The model under review builds one solid part; all positions refer to its coordinate system, in mm. A direction names the side the tool comes from. Coordinates: 2 decimals unless noted, no trailing zeros. Order: outer loops, then holes, each group sorted by start corner. A loop starts at its lowest first (then second) coordinate and runs counter-clockwise, first axis right, second up. Notation, with made-up numbers: (6, -6) -> (64, -6) arc R32 ccw to (64, 20) -> close; hole circle Ø9 at (-16.75, -18.5). An arc over 180 degrees is marked (long way). Use one line per item in the form item = value.
from build123d import *

# Parameters (mm, degrees)
HUB_DEPTH                         = 14
SKETCH4_R                         = 6
ARM_INSERT_1_DEPTH                = 30
SKETCH5_R                         = 6
ARM_INSERT_2_DEPTH                = 30
ARM_START                         = 30
SKETCH6_R                         = 6
ARM_INSERT_3_DEPTH                = 30
SKETCH7_R                         = 6
ARM_INSERT_4_DEPTH                = 30
SKETCH8_R                         = 8
HUB_LIGHTENING_HOLE_DEPTH         = 64.878932647
SKETCH9_R                         = 2.5
ARM_1_AND_3_LIGHTENING_HOLE_DEPTH = 100.535396168
SKETCH10_R                        = 2.5
ARM_2_AND_4_LIGHTENING_HOLE_DEPTH = 100.535396227


with BuildPart() as part:
    # Sketch1 → Hub (new body)
    with BuildSketch(Plane(origin=(0, 0, 0), x_dir=(1, 0, 0), z_dir=(0, 1, 0))):
        Polygon((14.071067812, 7), (14.071067812, -7), (7, -14.071067812), (-7, -14.071067812), (-14.071067812, -7), (-14.071067812, 7), (-7, 14.071067812), (7, 14.071067812), align=None)
    extrude(amount=HUB_DEPTH)

    # Sketch4 → Arm Insert 1 (add)
    with BuildSketch(Plane.XY.offset(14.071067812)):
        with Locations((0, 7)):
            Circle(SKETCH4_R)
    extrude(amount=ARM_INSERT_1_DEPTH)

    # Sketch5 → Arm Insert 2 (add)
    with BuildSketch(Plane(origin=(14.071067812, 0, 0), x_dir=(0, 0, -1), z_dir=(1, 0, 0))):
        with Locations((0, 7)):
            Circle(SKETCH5_R)
    extrude(amount=ARM_INSERT_2_DEPTH)

    # Sketch6 → Arm Insert 3 (add)
    with BuildSketch(Plane(origin=(0, 0, -14.071067812), x_dir=(-1, 0, 0), z_dir=(0, 0, -1)).offset(ARM_START)):
        with Locations(Location((0, 7, 0), (0, 0, 180))):
            Circle(SKETCH6_R)
    extrude(amount=-ARM_INSERT_3_DEPTH)

    # Sketch7 → Arm Insert 4 (add)
    with BuildSketch(Plane.ZY.offset(14.071067812).offset(ARM_START)):
        with Locations(Location((0, 7, 0), (0, 0, 180))):
            Circle(SKETCH7_R)
    extrude(amount=-ARM_INSERT_4_DEPTH)

    # Sketch8 → Hub Lightening Hole (cut, through all)
    with BuildSketch(Plane(origin=(0, 14, 0), x_dir=(1, 0, 0), z_dir=(0, 1, 0))):
        with Locations(Location((0, 0, 0), (0, 0, 270))):
            Circle(SKETCH8_R)
    extrude(amount=-HUB_LIGHTENING_HOLE_DEPTH, mode=Mode.SUBTRACT)

    # Sketch9 → Arm 1 and 3 Lightening Hole (cut, through all)
    with BuildSketch(Plane.XY.offset(44.071067812)):
        with Locations((0, 7)):
            Circle(SKETCH9_R)
    extrude(amount=-ARM_1_AND_3_LIGHTENING_HOLE_DEPTH, mode=Mode.SUBTRACT)

    # Sketch10 → Arm 2 and 4 Lightening Hole (cut, through all)
    with BuildSketch(Plane(origin=(44.071067812, 0, 0), x_dir=(0, 0, -1), z_dir=(1, 0, 0))):
        with Locations((0, 7)):
            Circle(SKETCH10_R)
    extrude(amount=-ARM_2_AND_4_LIGHTENING_HOLE_DEPTH, mode=Mode.SUBTRACT)


solid = part.part
Item 1: Draft analysis for pull direction Z (two halves, no side actions). For faces 5 (the face through (6, 0, -6)), 6 (the face through (-29.281, 5.198, -5.723)), 7 (the face through (-25.57, 4.56, 0.54)), state which applies: released by +Z, released by -Z, zero draft, split by the parting line, or undercut.
Results found:
face_5 = zero draft
face_6 = split by the parting line
face_7 = undercut
Item 2: To check wall thickness, follow L1, parallel to Y at x = 0, z = -18.5; L2, parallel to X at y = 10, z = 0; L3, parallel to Z at x = -30.5, y = 5.75. State the ranges of each line that lie inside material, in increasing order. Write a range as from..to.
Results found:
L1 = 1..4.5, 9.5..13
L2 = -44.07..-8, 8..44.07
L3 = -5.87..-2.17, 2.17..5.87
Item 3: We need section D-D (x = -20). Write out the cut boundary in (y, z), plus the area to 3 significant figures.
Results found:
outline = circle Ø12 at (7, 0); hole circle Ø5 at (7, 0)
area = 93.5 mm²
Item 4: We need section B-B (x = 0). Write out the cut boundary in (y, z).
Results found:
outline = (0, -14.07) -> (1, -14.07) -> (1, -44.07) -> (4.5, -44.07) -> (4.5, -8) -> (0, -8) -> close; (0, 8) -> (4.5, 8) -> (4.5, 44.07) -> (1, 44.07) -> (1, 14.07) -> (0, 14.07) -> close; (9.5, -44.07) -> (13, -44.07) -> (13, -14.07) -> (14, -14.07) -> (14, -8) -> (9.5, -8) -> close; (9.5, 8) -> (14, 8) -> (14, 14.07) -> (13, 14.07) -> (13, 44.07) -> (9.5, 44.07) -> close
Item 5: We need section A-A (z = 0). Write out the cut boundary in (x, y).
Results found:
outline = (-44.07, 1) -> (-14.07, 1) -> (-14.07, 0) -> (-8, 0) -> (-8, 4.5) -> (-44.07, 4.5) -> close; (-44.07, 9.5) -> (-8, 9.5) -> (-8, 14) -> (-14.07, 14) -> (-14.07, 13) -> (-44.07, 13) -> close; (8, 0) -> (14.07, 0) -> (14.07, 1) -> (44.07, 1) -> (44.07, 4.5) -> (8, 4.5) -> close; (8, 9.5) -> (44.07, 9.5) -> (44.07, 13) -> (14.07, 13) -> (14.07, 14) -> (8, 14) -> close
Item 6: We need section C-C (y = 11). Write out the cut boundary in (x, z), plus the area to 3 significant figures.
Results found:
outline = (-44.07, -4.47) -> (-14.07, -4.47) -> (-14.07, -7) -> (-7, -14.07) -> (-4.47, -14.07) -> (-4.47, -44.07) -> (4.47, -44.07) -> (4.47, -14.07) -> (7, -14.07) -> (14.07, -7) -> (14.07, -4.47) -> (44.07, -4.47) -> (44.07, 4.47) -> (14.07, 4.47) -> (14.07, 7) -> (7, 14.07) -> (4.47, 14.07) -> (4.47, 44.07) -> (-4.47, 44.07) -> (-4.47, 14.07) -> (-7, 14.07) -> (-14.07, 7) -> (-14.07, 4.47) -> (-44.07, 4.47) -> close; hole circle Ø16 at (0, 0)
area = 1,560 mm²
Item 7: Tool access review of faces 1 (the face through (5.723, 5.198, -29.281)), 2 (the face through (6.3, 6.9, 14.071)), 3 (the face through (28.86, 12.95, 0.78)), 4 (the face through (10.486, 6.902, -10.585)): name each direction out of +Z, -Z, +X, -X, +Y, -Y from which nothing blocks a thin tool from reaching the whole face with its end or side.
Results found:
face_1 = -Z
face_2 = +Z
face_3 = +X
face_4 = -Z, +X, +Y, -Y
Item 8: Clearance check with flat-ended pins moving along their axes: pin 1 (4.5 mm diameter, centred on x = 0, y = 7, fed in from -Z); pin 2 (1.5 mm diameter, centred on y = 9, z = 18, fed in from +X); pin 3 (5 mm diameter, centred on y = 2.5, z = -27.5, fed in from +X); pin 4 (4 mm diameter, centred on y = 12, z = 13.5, fed in from +X). State where each tip first meets the part, or that it passes through.
Results found:
pin_1 = through
pin_2 = 5.87
pin_3 = 5.66
pin_4 = 9.57
